The listing builds one solid part. Answer for the finished solid, in the listing's coordinates (mm). Face numbers are marked on the shaded views. Give positions to 0.01 mm unless a question says otherwise; leave off trailing zeros. Loops run counter-clockwise (first coordinate to the right, second up) from the corner with the lowest first, then second, coordinate; pieces in that order, holes last.
Item 1: Consider line 1 along Y through (x, z) = (0, 9) (3 decimals); line 2 along Y through (x, z) = (0, 6) (3 decimals); line 3 along Y through (x, z) = (0, 8.5) (3 decimals). Determine where each line is inside the solid, lowest interval first.
Item 2: Section B-B, the plane z = 12 is taken. Give the vertices of the cut face in (x, y) (3 decimals).
Item 3: Section C-C, the plane y = -24 is taken. Give the vertices of the cut face in (x, z), and give its area (3 significant figures).
Item 4: The mould has two halves that part along X. Classify the marked faces 1, 2 and 3: pulls with the +X half, pulls with the -X half, needs draft (parallel to the pull), parting line crosses it, or undercut.
Item 5: Section D-D, the plane x = 14.5 is taken. Give the vertices of the cut face in (y, z), and give its area (4 significant figures).
Item 6: Each of these flat-tipped pins is pushed along its axis until it touches: pin 1 Ø3 at (y, z) = (-16.5, 5) entering from +X; pin 2 Ø2 at (y, z) = (-16, 4.5) entering from -X; pin 3 Ø1 at (y, z) = (-10.5, 4.5) entering from -X; pin 4 Ø15 at (x, y) = (0, 0) entering from +Z. Where does it stop, or does it pass through?
Item 7: Section A-A, the plane z = 6.5 is taken. Give the vertices of the cut face in (x, y) (3 decimals).
from build123d import *

# Parameters (mm, degrees)
F0_R     = 28.575
F0_R_2   = 12.7
F1_DEPTH = 15.24
F2_SIZE2 = 0.3402954744
F2_SIZE  = 1.27
F4_D     = 3.4544
F4_DEPTH = 7.62
F4_TIP   = 1.0378064612


with BuildPart() as f1:
    # F0 (on Top) → F1 (new body)
    with BuildSketch(Plane.XY):
        Circle(F0_R)
        Circle(F0_R_2, mode=Mode.SUBTRACT)
    extrude(amount=F1_DEPTH)

    # F2
    f2_edges = [f1.edges().sort_by_distance(p)[0] for p in [
        (-12.7, 0, 15.24),
        (-12.7, 0, 0),
    ]]
    f2_side = f1.faces().sort_by_distance((-12.7, 0, 7.62))[0]
    chamfer(f2_edges, length=F2_SIZE, length2=F2_SIZE2, reference=f2_side)

    # F4
    with Locations(Plane(origin=(0, 0, 0), x_dir=(1, 0, 0), z_dir=(0, 0, -1))):
        with Locations((0, -19.685), (-19.685, 0), (0, 19.685), (19.685, 0)):
            Hole(F4_D / 2, depth=F4_DEPTH)
            with Locations((0, 0, -(F4_DEPTH + F4_TIP / 2))):  # 118° drill point
                Cone(0, F4_D / 2, F4_TIP, mode=Mode.SUBTRACT)


solid = f1.part
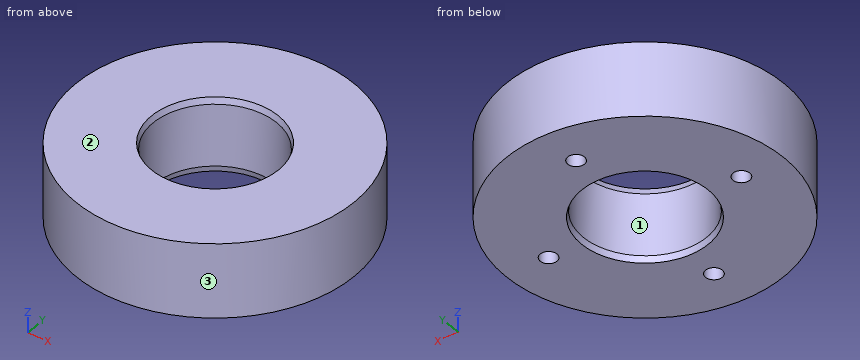
Worked answers:
1. line 1: y = -28.575 to -12.7, 12.7 to 28.575
1. line 2: y = -28.575 to -21.412, -17.958 to -12.7, 12.7 to 17.958, 21.412 to 28.575
1. line 3: y = -28.575 to -19.948, -19.422 to -12.7, 12.7 to 19.422, 19.948 to 28.575
2. outline: circle Ø57.15 at (0, 0); hole circle Ø25.4 at (0, 0)
3. outline: (-15.51, 0) - (15.51, 0) - (15.51, 15.24) - (-15.51, 15.24) - close
3. area: 473 mm2
4. face 1: undercut
4. face 2: needs draft
4. face 3: parting line crosses it
5. outline: (-24.62, 0) - (24.62, 0) - (24.62, 15.24) - (-24.62, 15.24) - close
5. area: 750.5 mm2
6. pin 1: stops at x = 24.32
6. pin 2: stops at x = -24.32
6. pin 3: stops at x = -26.77
6. pin 4: passes through
7. outline: circle Ø57.15 at (0, 0); hole circle Ø3.454 at (-19.685, 0); hole circle Ø25.4 at (0, 0); hole circle Ø3.454 at (0, -19.685); hole circle Ø3.454 at (0, 19.685); hole circle Ø3.454 at (19.685, 0)
